The model under review builds one solid part; all positions refer to its coordinate system, in mm. A direction names the side the tool comes from. Round coordinates to 2 decimals unless told otherwise and drop trailing zeros. Order: outer loops, then holes, each group sorted by start corner. A loop starts at its lowest first (then second) coordinate and runs counter-clockwise, first axis right, second up.
from build123d import *

# Parameters (mm, degrees)
ESQUISSE4_W                                      = 275
ESQUISSE4_H                                      = 157
BOSS_EXTRU_2_DEPTH                               = 4
FRAISAGE_POUR_VIS_T_TE_FRAIS_E_M42_AT_COUNT      = 2
FRAISAGE_POUR_VIS_T_TE_FRAIS_E_M42_AT_PITCH      = 235.512207752
FRAISAGE_POUR_VIS_T_TE_FRAIS_E_M42_2_COUNT       = 2
FRAISAGE_POUR_VIS_T_TE_FRAIS_E_M42_2_PITCH       = 229
FRAISAGE_POUR_VIS_T_TE_FRAIS_E_M42_3_COUNT       = 2
FRAISAGE_POUR_VIS_T_TE_FRAIS_E_M42_3_PITCH       = 55
CHAMBRAGE_POUR_VIS_T_TE_RONDE_6_PANS_D           = 6.6
CHAMBRAGE_POUR_VIS_T_TE_RONDE_6_PANS_CBORE_D     = 11.5
CHAMBRAGE_POUR_VIS_T_TE_RONDE_6_PANS_CBORE_DEPTH = 2
ESQUISSE9_W                                      = 219
ESQUISSE9_H                                      = 10
ESQUISSE9_H_2                                    = 39
ESQUISSE9_H_3                                    = 4
BOSS_EXTRU_3_DEPTH                               = 4


with BuildPart() as part:
    # Esquisse4 → Boss.-Extru.2 (new body)
    with BuildSketch(Plane.XY):
        Rectangle(ESQUISSE4_W, ESQUISSE4_H)
    extrude(amount=BOSS_EXTRU_2_DEPTH)

    # Esquisse6 → Fraisage pour vis à tête fraisée M42 (revolve, cut)
    with BuildSketch(Plane(origin=(-114.5, -21, 0), x_dir=(0, 1, 0), z_dir=(1, 0, 0))):
        Polygon((0, 0), (0, 4), (2.25, 4), (2.25, 2.45), (4.7, 0), align=None)
    fraisage_pour_vis_t_te_frais_e_m42 = revolve(axis=Axis((-114.5, -21, -6.35), (0, 0, 1)), mode=Mode.SUBTRACT)

    # Fraisage pour vis à tête fraisée M42 at: Fraisage pour vis à tête fraisée M42 ×2
    with Locations(*[Vector(0.972348747, 0.233533542, 0) * (i * FRAISAGE_POUR_VIS_T_TE_FRAIS_E_M42_AT_PITCH) for i in range(1, FRAISAGE_POUR_VIS_T_TE_FRAIS_E_M42_AT_COUNT)]):
        add(fraisage_pour_vis_t_te_frais_e_m42, mode=Mode.SUBTRACT)

    # Fraisage pour vis _ t_te frais_e M42 2: Fraisage pour vis à tête fraisée M42 ×2
    with Locations(*[(i * FRAISAGE_POUR_VIS_T_TE_FRAIS_E_M42_2_PITCH, 0, 0) for i in range(1, FRAISAGE_POUR_VIS_T_TE_FRAIS_E_M42_2_COUNT)]):
        add(fraisage_pour_vis_t_te_frais_e_m42, mode=Mode.SUBTRACT)

    # Fraisage pour vis _ t_te frais_e M42 3: Fraisage pour vis à tête fraisée M42 ×2
    with Locations(*[(0, i * FRAISAGE_POUR_VIS_T_TE_FRAIS_E_M42_3_PITCH, 0) for i in range(1, FRAISAGE_POUR_VIS_T_TE_FRAIS_E_M42_3_COUNT)]):
        add(fraisage_pour_vis_t_te_frais_e_m42, mode=Mode.SUBTRACT)

    # Chambrage pour Vis à tête ronde à 6 pans creux M61 (through all)
    with Locations(Plane.XY.offset(4)):
        with Locations((128.5, -69.5), (-128.5, -69.5), (-128.5, 69.5), (128.5, 69.5)):
            CounterBoreHole(CHAMBRAGE_POUR_VIS_T_TE_RONDE_6_PANS_D / 2, CHAMBRAGE_POUR_VIS_T_TE_RONDE_6_PANS_CBORE_D / 2, CHAMBRAGE_POUR_VIS_T_TE_RONDE_6_PANS_CBORE_DEPTH)

    # Esquisse9 → Boss.-Extru.3 (add)
    with BuildSketch(Plane.XY.offset(4)):
        with Locations((0, 34)):
            Rectangle(ESQUISSE9_W, ESQUISSE9_H)
        with Locations((0, 6.5)):
            Rectangle(ESQUISSE9_W, ESQUISSE9_H_2)
        with Locations((0, -21)):
            Rectangle(ESQUISSE9_W, ESQUISSE9_H)
        with Locations((0, -31)):
            Rectangle(ESQUISSE9_W, ESQUISSE9_H_3)
    extrude(amount=BOSS_EXTRU_3_DEPTH)


solid = part.part
(1) We need section D-D (x = -29). Give the boundary of the cut face in (y, z), and give its area (3 significant figures).
(2) The part is to be moulded in two halves that separate along X. For faces 3 (the cylindrical face through (-123.016, -67.773, 3.014)), 4 (the flat face through (-2, 34, 8)), say which applies: pulls with the +X half, pulls with the -X half, needs draft (parallel to the pull), parting line crosses it, or undercut.
(3) We need section C-C (y = 3). Give the boundary of the cut face in (x, z).
(4) Clearance check with flat-ended pins moving along their axes: P1, Ø3, axis at y = -22.5, z = 6, coming from the +X side; P2, Ø8, axis at x = 48, y = 49, coming from the +Z side; P3, Ø1.2, axis at x = 51.5, z = 6, coming from the -Y side. State where each tip first meets the part, or that it passes through.
(5) We need section B-B (x = -128.5). Give the boundary of the cut face in (y, z).
(6) We need section A-A (z = 5.5). Give the boundary of the cut face in (x, y), and give its area (3 significant figures).
(7) Tool access review of faces 1 (the cylindrical face through (130.93, 71.73, 0.99)), 2 (the cylindrical face through (133.984, -67.773, 3.014)): name each direction out of +Z, -Z, +X, -X, +Y, -Y from which nothing blocks a thin tool from reaching the whole face with its end or side.
(8) To check wall thickness, follow L1, parallel to X at y = 34, z = 3.4; L2, parallel to Y at x = 25, z = 6.25; L3, parallel to Y at x = -128.5, z = 2.95. State the ranges of each line that lie inside material, in increasing order.
Verdict:
1. outline: (-78.5, 0) - (78.5, 0) - (78.5, 4) - (39, 4) - (39, 8) - (29, 8) - (29, 4) - (26, 4) - (26, 8) - (-13, 8) - (-13, 4) - (-16, 4) - (-16, 8) - (-26, 8) - (-26, 4) - (-29, 4) - (-29, 8) - (-33, 8) - (-33, 4) - (-78.5, 4) - close
1. area: 880 mm2
2. face 3: undercut
2. face 4: needs draft
3. outline: (-137.5, 0) - (137.5, 0) - (137.5, 4) - (109.5, 4) - (109.5, 8) - (-109.5, 8) - (-109.5, 4) - (-137.5, 4) - close
4. P1: stops at x = 109.5
4. P2: stops at z = 4
4. P3: stops at y = -33
5. outline: (-78.5, 0) - (-72.8, 0) - (-72.8, 2) - (-75.25, 2) - (-75.25, 4) - (-78.5, 4) - close; (-66.2, 0) - (66.2, 0) - (66.2, 2) - (63.75, 2) - (63.75, 4) - (-63.75, 4) - (-63.75, 2) - (-66.2, 2) - close; (72.8, 0) - (78.5, 0) - (78.5, 4) - (75.25, 4) - (75.25, 2) - (72.8, 2) - close
6. outline: (-109.5, -33) - (109.5, -33) - (109.5, -29) - (-109.5, -29) - close; (-109.5, -26) - (109.5, -26) - (109.5, -16) - (-109.5, -16) - close; (-109.5, -13) - (109.5, -13) - (109.5, 26) - (-109.5, 26) - close; (-109.5, 29) - (109.5, 29) - (109.5, 39) - (-109.5, 39) - close
6. area: 13,800 mm2
7. face 1: +Z, -Z
7. face 2: +Z
8. L1: x = -137.5 to -116.75, -112.25 to 112.25, 116.75 to 137.5
8. L2: y = -33 to -29, -26 to -16, -13 to 26, 29 to 39
8. L3: y = -78.5 to -75.25, -63.75 to 63.75, 75.25 to 78.5
